Autodesk Inventor part; units mm, degrees
ref_plane "YZ Plane" through (0, 0, 0) normal (1, 0, 0) x (0, 1, 0)
ref_plane "XZ Plane" through (0, 0, 0) normal (0, 1, 0) x (-1, 0, 0)
ref_plane "XY Plane" through (0, 0, 0) normal (0, 0, 1) x (1, 0, 0)
sketch "스케치1" plane through (0, 0, 0) normal (0, 0, 1) x (1, 0, 0)
  circle A0 centre (0, 0) radius 60 construction
  line L0 (0, 0) -> (0, 95.3997)
  line L1 (0, 0) -> (-132.5472, 0)
  line L2 (52.5, 52.5) -> (-52.5, 52.5)
  line L3 (-52.5, 52.5) -> (-52.5, -52.5)
  line L4 (-52.5, -52.5) -> (52.5, -52.5)
  line L5 (52.5, -52.5) -> (52.5, 52.5)
  line L6 (52.5, 52.5) -> (-52.5, -52.5) construction
  line L7 (-52.5, 52.5) -> (52.5, -52.5) construction
  arc A1 (-46.6369, 65) -> (-46.6369, -65) centre (0, 0) ccw
  arc A2 (46.6369, -65) -> (46.6369, 65) centre (0, 0) ccw
  line L8 (-46.6369, 65) -> (46.6369, 65)
  line L9 (-46.6369, -65) -> (46.6369, -65)
  line L10 (0, 0) -> (104.7447, 43.3867)
  line L11 (0, 0) -> (113.3748, 0) construction
  circle A3 centre (55.4328, 22.961) radius 1.5
  dimension "d0" = 120
  dimension "d49" = 105
  dimension "d50" = 105
  dimension "d56" = 22.5
  dimension "d57" = 3
extrude "돌출1" add sketch "스케치1" along normal blind 1
sketch "스케치5" plane through (0, 0, 1) normal (0, 0, 1) x (1, 0, 0)
  arc A0 (46.6369, -65) -> (46.6369, 65) centre (0, 0) ccw
  circle A1 centre (55.4328, 22.961) radius 1.5
  circle A2 centre (55.4328, 22.961) radius 1.5
  circle A3 centre (22.961, 55.4328) radius 1.5
  circle A4 centre (-22.961, 55.4328) radius 1.5
  circle A5 centre (-55.4328, 22.961) radius 1.5
  circle A6 centre (-55.4328, -22.961) radius 1.5
  circle A7 centre (-22.961, -55.4328) radius 1.5
  circle A8 centre (22.961, -55.4328) radius 1.5
  circle A9 centre (55.4328, -22.961) radius 1.5
  dimension "d60" = 360
extrude "돌출5" cut sketch "스케치5" against normal through all
sketch "스케치6" plane through (0, 0, 1) normal (0, 0, 1) x (1, 0, 0)
  arc A0 (-46.6369, 65) -> (-46.6369, -65) centre (0, 0) ccw
  line L0 (36.5, 36.5) -> (-36.5, 36.5) construction
  line L1 (-36.5, 36.5) -> (-36.5, -36.5) construction
  line L2 (-36.5, -36.5) -> (36.5, -36.5) construction
  line L3 (36.5, -36.5) -> (36.5, 36.5) construction
  line L4 (36.5, 36.5) -> (-36.5, -36.5) construction
  line L5 (-36.5, 36.5) -> (36.5, -36.5) construction
  circle A1 centre (-36.5, 36.5) radius 1.5
  dimension "d64" = 73
  dimension "d65" = 73
  dimension "d66" = 3
extrude "돌출6" cut sketch "스케치6" against normal through all
pattern_circular "원형 패턴1" count 4 over 360 about axis through (0, 0, 0) along (0, 0, 1) of "돌출6"
sketch "스케치7" plane through (0, 0, 1) normal (0, 0, 1) x (1, 0, 0)
  arc A0 (-46.6369, 65) -> (-46.6369, -65) centre (0, 0) ccw
  line L0 (52.5, 52.5) -> (-52.5, 52.5) construction
  line L1 (-52.5, 52.5) -> (-52.5, -52.5) construction
  line L2 (-52.5, -52.5) -> (52.5, -52.5) construction
  line L3 (52.5, -52.5) -> (52.5, 52.5) construction
  line L4 (52.5, 52.5) -> (-52.5, -52.5) construction
  line L5 (-52.5, 52.5) -> (52.5, -52.5) construction
  circle A1 centre (-52.5, 52.5) radius 2.5
  dimension "d72" = 105
  dimension "d73" = 105
  dimension "d74" = 5
extrude "돌출7" cut sketch "스케치7" against normal through all
pattern_circular "원형 패턴2" count 4 over 360 about axis through (0, 0, 0) along (0, 0, 1) of "돌출7"
sketch "스케치9" plane through (0, 0, 1) normal (0, 0, 1) x (1, 0, 0)
  arc A0 (-46.6369, 65) -> (-46.6369, -65) centre (0, 0) ccw
  line L0 (-34.8236, -59) -> (-59, -34.8236)
  line L1 (-59, -34.8236) -> (-59, 34.8236)
  line L2 (-59, 34.8236) -> (-34.8236, 59)
  line L3 (-34.8236, 59) -> (34.8236, 59)
  line L4 (34.8236, 59) -> (59, 34.8236)
  line L5 (59, 34.8236) -> (59, -34.8236)
  line L6 (59, -34.8236) -> (34.8236, -59)
  line L7 (34.8236, -59) -> (-34.8236, -59)
  circle A1 centre (52.5, -52.5) radius 2.5
  circle A2 centre (-52.5, 52.5) radius 2.5
  circle A3 centre (-52.5, -52.5) radius 2.5
  circle A4 centre (52.5, 52.5) radius 2.5
  line L8 (-84.5, -70.75) -> (65.5, -70.75)
  line L9 (65.5, -70.75) -> (65.5, 70.75)
  line L10 (65.5, 70.75) -> (-84.5, 70.75)
  line L11 (-84.5, 70.75) -> (-84.5, -70.75)
  circle A5 centre (0, 0) radius 45
  dimension "d80" = 90
extrude "돌출8" cut sketch "스케치9" against normal through all contours A5
sketch "스케치11" plane through (0, 0, 1) normal (0, 0, 1) x (1, 0, 0)
  line L0 (65.5, -70.75) -> (65.5, 70.75)
  line L1 (65.5, 70.75) -> (105.9964, 70.75)
  line L2 (105.9964, 70.75) -> (105.9964, -90.2742)
  line L3 (105.9964, -90.2742) -> (65.5, -90.2742)
  line L4 (65.5, -90.2742) -> (65.5, 70.75)
extrude "돌출9" cut sketch "스케치11" against normal through all
mirror "미러3" about plane through (0, 0, 0) normal (1, 0, 0) of "돌출9"
fillet "모깎기3" radius 33.75 4 edges at (65.5, 45.932, 0.5) (65.5, -45.932, 0.5) (-65.5, -45.932, 0.5) (-65.5, 45.932, 0.5)
properties part number "모터드라이버 지지대 철판가공"
For this review, take the finished solid that the model builds, in its own axes (mm). Coordinates: 2 decimals unless noted, no trailing zeros. Order: outer loops, then holes, each group sorted by start corner. A loop starts at its lowest first (then second) coordinate and runs counter-clockwise, first axis right, second up. Notation, with made-up numbers: (12, 50.5) -> (66, 50.5) arc R22 ccw to (66, 78.5) -> close; hole circle Ø9 at (61, 54.5). An arc over 180 degrees is marked (long way). Answer as CSV lines item,"result".
Q1. Draft analysis for pull direction X (two halves, no side actions). For faces 1 (the face through (-50.19, 51.54, 0.51)), 2 (the face through (-15, 44, 0)), 3 (the face through (-24.07, -54.42, 0.51)), 4 (the face through (50.951, -61.677, 0.493)), state which applies: released by +X, released by -X, zero draft, split by the parting line, or undercut.
Model answer:
face 1,"undercut"
face 2,"zero draft"
face 3,"undercut"
face 4,"released by +X"
Q2. Wall thickness on line 1 along Y through (x, z) = (-1.5, 0.3) (3 decimals); line 2 along Y through (x, z) = (-52.5, 0.7); line 3 along Y through (x, z) = (-15.5, 0.55): over which ranges is each line inside the solid? List them lowest first. Write a range as [from, to].
Model answer:
line 1,"y = [-65, -44.975], [44.975, 65]"
line 2,"y = [-60.36, -55], [-50, 50], [55, 60.36]"
line 3,"y = [-65, -42.25], [42.25, 65]"
Q3. We need section D-D (x = 36.5). State the section outline as (y, z) points, plus the area to 3 significant figures.
Model answer:
outline,"(-65, 0) -> (-38, 0) -> (-38, 1) -> (-65, 1) -> close; (-35, 0) -> (-26.32, 0) -> (-26.32, 1) -> (-35, 1) -> close; (26.32, 0) -> (35, 0) -> (35, 1) -> (26.32, 1) -> close; (38, 0) -> (65, 0) -> (65, 1) -> (38, 1) -> close"
area,"71.4 mm2"
Q4. We need section A-A (y = -43). State the section outline as (x, z) points.
Model answer:
outline,"(-64.17, 0) -> (-13.27, 0) -> (-13.27, 1) -> (-64.17, 1) -> close; (13.27, 0) -> (64.17, 0) -> (64.17, 1) -> (13.27, 1) -> close"
Q5. We need section C-C (z = 0.15). Count the separate pieces of the cut face and the enclosed holes in it, plus the area to 3 significant figures.
Model answer:
separate pieces,"1"
enclosed holes,"17"
area,"9,790 mm2"
Q6. We need section B-B (x = 0). State the section outline as (y, z) points.
Model answer:
outline,"(-65, 0) -> (-45, 0) -> (-45, 1) -> (-65, 1) -> close; (45, 0) -> (65, 0) -> (65, 1) -> (45, 1) -> close"
Q7. Clearance check with a flat-ended pin moving along its axis: pin 1 Ø2.5 at (x, y) = (22.96, -55.43) entering from -Z. State where the tip first meets the part, or that it passes through.
Model answer:
pin 1,"passes through"
